from build123d import *

# Parameters (mm, degrees)
ESQUISSE1_W             = 32
ESQUISSE1_H             = 32
BOSS_EXTRU_1_DEPTH      = 1.5
ESQUISSE2_R             = 10.05
ESQUISSE2_R_2           = 9.95
ENL_V_MAT_EXTRU_1_DEPTH = 0.2
ESQUISSE3_R             = 0.25
ENL_V_MAT_EXTRU_2_DEPTH = 2.5
ESQUISSE4_W             = 31
ESQUISSE4_H             = 31
ENL_V_MAT_EXTRU_3_DEPTH = 0.1
ENL_V_MAT_EXTRU_4_DEPTH = 0.1


with BuildPart() as part:
    # Esquisse1 → Boss.-Extru.1 (new body)
    with BuildSketch(Plane.XY):
        Rectangle(ESQUISSE1_W, ESQUISSE1_H)
    extrude(amount=BOSS_EXTRU_1_DEPTH)

    # Esquisse2 → Enlèv. mat.-Extru.1 (cut)
    with BuildSketch(Plane(origin=(0, 0, 0), x_dir=(-1, 0, 0), z_dir=(0, 0, -1))):
        Circle(ESQUISSE2_R)
        Circle(ESQUISSE2_R_2, mode=Mode.SUBTRACT)
    extrude(amount=-ENL_V_MAT_EXTRU_1_DEPTH, mode=Mode.SUBTRACT)

    # Esquisse3 → Enlèv. mat.-Extru.2 (cut, through all)
    with BuildSketch(Plane(origin=(0, 0, 0), x_dir=(-1, 0, 0), z_dir=(0, 0, -1))):
        with Locations((0, 10.5)):
            Circle(ESQUISSE3_R)
        with Locations((4.01817604, 9.700735091)):
            Circle(ESQUISSE3_R)
        with Locations((7.424621202, 7.424621202)):
            Circle(ESQUISSE3_R)
        with Locations((9.700735091, 4.01817604)):
            Circle(ESQUISSE3_R)
        with Locations((10.5, 0)):
            Circle(ESQUISSE3_R)
        with Locations((9.700735091, -4.01817604)):
            Circle(ESQUISSE3_R)
        with Locations((7.424621202, -7.424621202)):
            Circle(ESQUISSE3_R)
        with Locations((4.01817604, -9.700735091)):
            Circle(ESQUISSE3_R)
        with Locations((0, -10.5)):
            Circle(ESQUISSE3_R)
        with Locations((-4.01817604, -9.700735091)):
            Circle(ESQUISSE3_R)
        with Locations((-7.424621202, -7.424621202)):
            Circle(ESQUISSE3_R)
        with Locations((-9.700735091, -4.01817604)):
            Circle(ESQUISSE3_R)
        with Locations((-10.5, 0)):
            Circle(ESQUISSE3_R)
        with Locations((-9.700735091, 4.01817604)):
            Circle(ESQUISSE3_R)
        with Locations((-7.424621202, 7.424621202)):
            Circle(ESQUISSE3_R)
        with Locations((-4.01817604, 9.700735091)):
            Circle(ESQUISSE3_R)
    extrude(amount=-ENL_V_MAT_EXTRU_2_DEPTH, mode=Mode.SUBTRACT)

    # Esquisse4 → Enlèv. mat.-Extru.3 (cut)
    with BuildSketch(Plane(origin=(0, 0, 0), x_dir=(-1, 0, 0), z_dir=(0, 0, -1))):
        Rectangle(ESQUISSE4_W, ESQUISSE4_H)
    extrude(amount=-ENL_V_MAT_EXTRU_3_DEPTH, mode=Mode.SUBTRACT)

    # Esquisse5 → Enlèv. mat.-Extru.4 (cut)
    with BuildSketch(Plane.XY.offset(1.5)):
        with BuildLine():
            Line((-3, 3), (3, 3))
            Line((3, 3), (3, 1))
            Line((3, 1), (1.5, 1))
            ThreePointArc((1.5, 1), (0, 1.802775638), (-1.5, 1))
            Line((-1.5, 1), (-3, 1))
            Line((-3, 1), (-3, 3))
        make_face()
        with BuildLine():
            Line((-3, -3), (-3, -1))
            Line((-3, -1), (-1.5, -1))
            ThreePointArc((-1.5, -1), (0, -1.802775638), (1.5, -1))
            Line((1.5, -1), (3, -1))
            Line((3, -1), (3, -3))
            Line((3, -3), (-3, -3))
        make_face()
    extrude(amount=-ENL_V_MAT_EXTRU_4_DEPTH, mode=Mode.SUBTRACT)


solid = part.part
Part model, mm, in its own coordinate system. A direction names the side the tool comes from. Coordinates: 2 decimals unless noted, no trailing zeros. Write each loop counter-clockwise with the first axis right and the second up, starting at its lowest first coordinate (ties: lowest second). Pieces come first, ordered by that corner, then holes. Notation, with made-up numbers: M 44.5,-35.75 L 50.5,-35.75 A13 cw 50.5,-21.75 Z; hole C 69.5,29 d3. An arc over 180 degrees is marked long. Return JSON: item names as keys, results as strings.
1. Pull direction X, two halves, no side cores. Call faces 4 (the face through (0, 0, 1.5)), 5 (the face through (-3, -10, 0.1)), 6 (the face through (16, 0, 1)): pulls with the +X half, pulls with the -X half, needs draft (parallel to the pull), parting line crosses it, or undercut.
Determined:
{"face 4": "needs draft", "face 5": "undercut", "face 6": "pulls with the +X half"}
2. Saw through at C-C, the plane y = 5.5. Write the cut outline in (x, z).
Determined:
{"outline": "M -16,0 L -15.5,0 L -15.5,0.1 L -8.41,0.1 L -8.41,0.2 L -8.29,0.2 L -8.29,0.1 L 8.29,0.1 L 8.29,0.2 L 8.41,0.2 L 8.41,0.1 L 15.5,0.1 L 15.5,0 L 16,0 L 16,1.5 L -16,1.5 Z"}
3. Saw through at B-B, the plane x = -2. Write the cut outline in (y, z).
Determined:
{"outline": "M -16,0 L -15.5,0 L -15.5,0.1 L -9.85,0.1 L -9.85,0.2 L -9.75,0.2 L -9.75,0.1 L 9.75,0.1 L 9.75,0.2 L 9.85,0.2 L 9.85,0.1 L 15.5,0.1 L 15.5,0 L 16,0 L 16,1.5 L 3,1.5 L 3,1.4 L 1,1.4 L 1,1.5 L -1,1.5 L -1,1.4 L -3,1.4 L -3,1.5 L -16,1.5 Z"}
4. 3-axis set-ups, long thin cutter, end or side, ignore diameter. For faces 1 (the face through (0, 0, 0.1)), 2 (the face through (0, -16, 1)), 3 (the face through (0, 2, 1.4)): which of +Z, -Z, +X, -X, +Y, -Y reach the whole face in a straight line?
Determined:
{"face 1": "-Z", "face 2": "+Z, -Z, +X, -X, -Y", "face 3": "+Z"}
5. Flat gauge pins, fed straight in: pin 1 Ø5 at (x, y) = (10.5, 2.5) entering from -Z; pin 2 Ø0.6 at (x, y) = (0, 2.5) entering from +Z. Where does each tip first touch, or does it go through?
Determined:
{"pin 1": "z = 0.1", "pin 2": "z = 1.4"}
6. Probe L1, parallel to Y at x = 0, z = 1.1; L2, parallel to X at y = 4, z = 0.3; L3, parallel to Y at x = -10.5, z = 1.1. List the from-to ranges inside material, lowest first.
Determined:
{"L1": "-16 to -10.75, -10.25 to 10.25, 10.75 to 16", "L2": "-16 to -9.95, -9.45 to 9.45, 9.95 to 16", "L3": "-16 to -0.25, 0.25 to 16"}
7. Saw through at A-A, the plane y = 11.5. Write the cut outline in (x, z).
Determined:
{"outline": "M -16,0 L -15.5,0 L -15.5,0.1 L 15.5,0.1 L 15.5,0 L 16,0 L 16,1.5 L -16,1.5 Z"}
